```python
from build123d import *

# Parameters (mm, degrees)
SKETCH1_W           = 200
SKETCH1_H           = 125
BOSS_EXTRUDE1_DEPTH = 120
BOSS_EXTRUDE2_DEPTH = 120
SKETCH3_W           = 200
SKETCH3_H           = 125
CUT_EXTRUDE1_DEPTH  = 120
FILLET1_R           = 5
SKETCH4_W           = 100
SKETCH4_H           = 40
BOSS_EXTRUDE3_DEPTH = 100
FILLET3_R           = 3
SKETCH5_W           = 190
SKETCH5_H           = 115
CUT_EXTRUDE2_DEPTH  = 115
SKETCH6_W           = 15
SKETCH6_H           = 15
BOSS_EXTRUDE4_DEPTH = 110
SKETCH7_W           = 200
SKETCH7_H           = 100
BOSS_EXTRUDE5_DEPTH = 40
FILLET4_R           = 20
SKETCH9_W           = 189.724209099
SKETCH9_H           = 80
CUT_EXTRUDE9_DEPTH  = 35
CUT_EXTRUDE10_DEPTH = 35
CUT_EXTRUDE11_DEPTH = 20
FILLET5_R           = 2
SKETCH11_R          = 5
CUT_EXTRUDE12_DEPTH = 132


with BuildPart() as part:
    # Sketch1 → Boss-Extrude1 (new body)
    with BuildSketch(Plane(origin=(0, 0, 0), x_dir=(1, 0, 0), z_dir=(0, 1, 0))):
        with Locations((8.778519755, -18.055555556)):
            Rectangle(SKETCH1_W, SKETCH1_H)
    extrude(amount=BOSS_EXTRUDE1_DEPTH)

    # Sketch2 → Boss-Extrude2 (add)
    with BuildSketch(Plane(origin=(0, 120, 0), x_dir=(1, 0, 0), z_dir=(0, 1, 0))):
        with BuildLine():
            Line((-86.221480245, 44.444444444), (103.778519755, 44.444444444))
            ThreePointArc((103.778519755, 44.444444444), (107.314053661, 42.97997835), (108.778519755, 39.444444444))
            Line((108.778519755, 39.444444444), (108.778519755, -75.555555556))
            ThreePointArc((108.778519755, -75.555555556), (107.314053661, -79.091089461), (103.778519755, -80.555555556))
            Line((103.778519755, -80.555555556), (-86.221480245, -80.555555556))
            ThreePointArc((-86.221480245, -80.555555556), (-89.757014151, -79.091089461), (-91.221480245, -75.555555556))
            Line((-91.221480245, -75.555555556), (-91.221480245, 39.444444444))
            ThreePointArc((-91.221480245, 39.444444444), (-89.757014151, 42.97997835), (-86.221480245, 44.444444444))
        make_face()
    extrude(amount=BOSS_EXTRUDE2_DEPTH)

    # Sketch3 → Cut-Extrude1 (cut)
    with BuildSketch(Plane(origin=(0, 0, 0), x_dir=(-1, 0, 0), z_dir=(0, -1, 0))):
        with Locations((-8.778519755, -18.055555556)):
            Rectangle(SKETCH3_W, SKETCH3_H)
    extrude(amount=-CUT_EXTRUDE1_DEPTH, mode=Mode.SUBTRACT)

    # Fillet1
    fillet1_edges = [part.edges().sort_by_distance(p)[0] for p in [
        (-89.757014151, 240, -42.97997835),
        (-91.221480245, 240, 18.055555556),
        (-89.757014151, 240, 79.091089461),
        (8.778519755, 240, 80.555555556),
        (107.314053661, 240, 79.091089461),
        (108.778519755, 240, 18.055555556),
        (107.314053661, 240, -42.97997835),
        (8.778519755, 240, -44.444444444),
    ]]
    fillet(fillet1_edges, radius=FILLET1_R)

    # Sketch4 → Boss-Extrude3 (add)
    with BuildSketch(Plane(origin=(108.778519755, 0, 0), x_dir=(0, 0, -1), z_dir=(1, 0, 0))):
        with Locations((-18.055555556, 140)):
            Rectangle(SKETCH4_W, SKETCH4_H)
    extrude(amount=BOSS_EXTRUDE3_DEPTH)

    # Fillet3
    fillet3_edges = [part.edges().sort_by_distance(p)[0] for p in [
        (158.778519755, 160, 68.055555556),
        (158.778519755, 160, -31.944444444),
    ]]
    fillet(fillet3_edges, radius=FILLET3_R)

    # Sketch5 → Cut-Extrude2 (cut)
    with BuildSketch(Plane(origin=(0, 120, 0), x_dir=(-1, 0, 0), z_dir=(0, -1, 0))):
        with Locations((-8.778519755, -18.055555556)):
            Rectangle(SKETCH5_W, SKETCH5_H)
    extrude(amount=-CUT_EXTRUDE2_DEPTH, mode=Mode.SUBTRACT)

    # Sketch6 → Boss-Extrude4 (add)
    with BuildSketch(Plane(origin=(0, 235, 0), x_dir=(-1, 0, 0), z_dir=(0, -1, 0))):
        with Locations((78.721480245, -68.055555556)):
            Rectangle(SKETCH6_W, SKETCH6_H)
        with Locations((-96.278519755, -68.055555556)):
            Rectangle(SKETCH6_W, SKETCH6_H)
        with Locations((-96.278519755, 31.944444444)):
            Rectangle(SKETCH6_W, SKETCH6_H)
        with Locations((78.721480245, 31.944444444)):
            Rectangle(SKETCH6_W, SKETCH6_H)
    extrude(amount=BOSS_EXTRUDE4_DEPTH)

    # Sketch7 → Boss-Extrude5 (add)
    with BuildSketch(Plane(origin=(208.778519755, 0, 0), x_dir=(0, 0, -1), z_dir=(1, 0, 0))):
        with Locations((-18.055555556, 170)):
            Rectangle(SKETCH7_W, SKETCH7_H)
    extrude(amount=BOSS_EXTRUDE5_DEPTH)

    # Fillet4
    fillet4_edges = [part.edges().sort_by_distance(p)[0] for p in [
        (228.778519755, 220, 118.055555556),
        (228.778519755, 220, -81.944444444),
    ]]
    fillet(fillet4_edges, radius=FILLET4_R)

    # Sketch9 → Cut-Extrude9 (cut)
    with BuildSketch(Plane(origin=(248.778519755, 0, 0), x_dir=(0, 0, -1), z_dir=(1, 0, 0))):
        with Locations((-17.917660106, 160)):
            Rectangle(SKETCH9_W, SKETCH9_H)
    extrude(amount=-CUT_EXTRUDE9_DEPTH, mode=Mode.SUBTRACT)

    # Sketch9<3> → Cut-Extrude10 (cut)
    with BuildSketch(Plane(origin=(248.778519755, 0, 0), x_dir=(0, 0, -1), z_dir=(1, 0, 0))):
        with BuildLine():
            Line((-112.779764655, 200), (76.944444444, 200))
            ThreePointArc((76.944444444, 200), (72.551046162, 210.606601718), (61.944444444, 215))
            Line((61.944444444, 215), (-98.055555556, 214.7242091))
            ThreePointArc((-98.055555556, 214.7242091), (-108.467143658, 210.411588102), (-112.779764655, 200))
        make_face()
    extrude(amount=-CUT_EXTRUDE10_DEPTH, mode=Mode.SUBTRACT)

    # Sketch10 → Cut-Extrude11 (cut)
    with BuildSketch(Plane(origin=(108.778519755, 0, 0), x_dir=(0, 0, -1), z_dir=(1, 0, 0))):
        with BuildLine():
            Line((-28.055555556, 222), (-28.055555556, 172))
            ThreePointArc((-28.055555556, 172), (-18.055555556, 162), (-8.055555556, 172))
            Line((-8.055555556, 172), (-8.055555556, 222))
            ThreePointArc((-8.055555556, 222), (-18.055555556, 232), (-28.055555556, 222))
        make_face()
    extrude(amount=-CUT_EXTRUDE11_DEPTH, mode=Mode.SUBTRACT)

    # Fillet5
    fillet5_edges = [part.edges().sort_by_distance(p)[0] for p in [
        (108.778519755, 232, 18.055555556),
        (108.778519755, 197, 28.055555556),
        (108.778519755, 162, 18.055555556),
        (108.778519755, 197, 8.055555556),
    ]]
    fillet(fillet5_edges, radius=FILLET5_R - 0.0001)  # a hair under: the kernel refuses the full size

    # Sketch11 → Cut-Extrude12 (cut)
    with BuildSketch(Plane(origin=(213.778519755, 0, 0), x_dir=(0, 0, -1), z_dir=(1, 0, 0))):
        with Locations((-42.779764655, 140)):
            Circle(SKETCH11_R)
        with Locations((6.944444444, 140)):
            Circle(SKETCH11_R)
    extrude(amount=-CUT_EXTRUDE12_DEPTH, mode=Mode.SUBTRACT)


solid = part.part
```
The model under review builds one solid part; all positions refer to its coordinate system, in mm. A direction names the side the tool comes from. Round coordinates to 2 decimals unless told otherwise and drop trailing zeros. Write each loop counter-clockwise with the first axis right and the second up, starting at its lowest first coordinate (ties: lowest second). Pieces come first, ordered by that corner, then holes. Notation, with made-up numbers: (59, 24) - (97, 24) arc R29 ccw to (97, 54) - close; hole circle Ø5 at (70.25, 73.25). An arc over 180 degrees is marked (long way). Use one line per item in the form item = value.
Q1. Consider section A-A (x = 118.5). State the section outline as (y, z) points, and give its area (3 significant figures).
Answer key:
outline = (120, -31.94) - (157, -31.94) arc R3 ccw to (160, -28.94) - (160, 65.06) arc R3 ccw to (157, 68.06) - (120, 68.06) - close; hole circle Ø10 at (140, -6.94); hole circle Ø10 at (140, 42.78)
area = 3,840 mm2
Q2. Draft analysis for pull direction X (two halves, no side actions). For faces 1 (the flat face through (10, 235, 17)), 2 (the flat face through (228, 159, -81.944)), 3 (the flat face through (-91.221, 177, 19)), state which applies: +X half, -X half, draft (parallel to the pull), parting line (faces both ways), or undercut.
Answer key:
face_1 = undercut
face_2 = draft
face_3 = -X half
Q3. Consider section C-C (x = 73.5). State the section outline as (y, z) points.
Answer key:
outline = (120, -44.44) - (235, -44.44) arc R5 ccw to (240, -39.44) - (240, 75.56) arc R5 ccw to (235, 80.56) - (120, 80.56) - (120, 75.56) - (235, 75.56) - (235, -39.44) - (120, -39.44) - close
Q4. Tool access review of faces 4 (the flat face through (158, 138, 68.056)), 5 (the flat face through (228, 220, 19)), 6 (the cylindrical face through (159.549, 135.564, 40.473)), 7 (the flat face through (-71.221, 181, 68)): name each direction out of +Z, -Z, +X, -X, +Y, -Y from which nothing blocks a thin tool from reaching the whole face with its end or side.
Answer key:
face_4 = +Z, +Y, -Y
face_5 = +Z, -Z, +X, +Y
face_6 = +X
face_7 = -Y
Q5. For line 1 (X direction, y = 155, z = -38); line 2 (X direction, y = 214.5, z = 55.5); line 3 (Z direction, x = -29.5, y = 188), list the stretches that pass through material, from the lowest coordinate up. Write a range as [from, to].
Answer key:
line_1 = [-91.22, -71.22], [88.78, 108.78], [208.78, 213.78]
line_2 = [-91.22, -86.22], [103.78, 108.78], [208.78, 213.78]
line_3 = [-44.44, -39.44], [75.56, 80.56]
Q6. Insertion check: pin 1 Ø10 at (x, z) = (-14, 47) entering from -Y; pin 2 Ø4.5 at (x, y) = (98, 190.5) entering from -Z; pin 3 Ø0.9 at (x, y) = (105.5, 187.5) entering from +Z. Each pin has a flat end and moves straight along its axis. Give the tip position at first contact, or say it passes through.
Answer key:
pin_1 = 235
pin_2 = -44.44
pin_3 = 80.39
